Input: part model. Units: mm. Frame: model coordinates. Face numbers are marked on the shaded views. A direction names the side the tool comes from. Round coordinates to 2 decimals unless told otherwise and drop trailing zeros. Loops run counter-clockwise (first coordinate to the right, second up) from the corner with the lowest first, then second, coordinate; pieces in that order, holes last. Notation, with made-up numbers: (18.5, -19) -> (42.5, -19) arc R23 cw to (42.5, -8) -> close; hole circle Ø1 at (-39.5, 25). An arc over 180 degrees is marked (long way). One line per question, with ' | ' between items. Start each with the question number.
Q1. Material intervals for L1, parallel to X at y = 0, z = 32.1; L2, parallel to X at y = 0, z = 27.5; L3, parallel to X at y = 3.25, z = 28, sorted ascending.
Q2. Mould query, pull axis X, two halves, no side actions, for the marked faces 4, 5 and 6. Classes: pulls with the +X half, pulls with the -X half, needs draft (parallel to the pull), parting line crosses it, or undercut.
Q3. Contact query for flat-ended pins moving along their axis: P1, Ø9, axis at x = -34, y = 1.5, coming from the -Z side; P2, Ø6, axis at y = 3.5, z = 11, coming from the -X side; P3, Ø1, axis at x = 8.5, y = -0.5, coming from the +Z side; P4, Ø4, axis at x = -30.5, z = 19.5, coming from the +Y side. Output: stop coordinate, or through.
Q4. Access query for the marked faces 1, 2 and 3. Directions: +Z, -Z, +X, -X, +Y, -Y. A direction counts if a zero-diameter tool reaches every point of the face in a straight line with its end or side. Return the directions, or none.
Q5. Cut plane A-A on y = -5. Return loops of the section in (x, z), and give its area (3 significant figures).
Q6. Cut plane B-B on z = 14.5. Return loops of the section in (x, y), and give its area (3 significant figures).
Q7. Cut plane C-C on y = 0. State how many separate pieces and enclosed holes the cut face has, and give its area (3 significant figures).
Autodesk Inventor part; units mm, degrees
ref_plane "YZ Plane" through (0, 0, 0) normal (1, 0, 0) x (0, 1, 0)
ref_plane "XZ Plane" through (0, 0, 0) normal (0, 1, 0) x (-1, 0, 0)
ref_plane "XY Plane" through (0, 0, 0) normal (0, 0, 1) x (1, 0, 0)
sketch "Sketch1" plane through (0, 0, 0) normal (0, 0, 1) x (1, 0, 0)
  line L0 (-38.9875, 7.874) -> (38.9875, 7.874)
  line L1 (38.9875, 7.874) -> (38.9875, -7.874)
  line L2 (38.9875, -7.874) -> (-38.9875, -7.874)
  line L3 (-38.9875, -7.874) -> (-38.9875, 7.874)
  point P0 (0, 0)
  dimension "d2" = 77.975
  dimension "d3" = 38.9875
  dimension "d6" = 15.748
  dimension "d7" = 7.874
extrude "Extrusion1" add sketch "Sketch1" along normal blind 33.1075
sketch "Sketch2" plane through (0, 0, 0) normal (0, 0, -1) x (-1, 0, 0)
  line L0 (38.9875, 7.874) -> (38.9875, -7.874)
  line L1 (-38.9875, -7.874) -> (-38.9875, 7.874)
  line L2 (38.9875, -7.874) -> (-38.9875, -7.874)
  line L3 (-38.9875, 7.874) -> (38.9875, 7.874)
  line L4 (38.9875, -7.874) -> (26.9875, -7.874)
  line L5 (26.9875, -7.874) -> (26.9875, 7.874)
  line L6 (26.9875, 7.874) -> (38.9875, 7.874)
  line L7 (38.9875, 7.874) -> (38.9875, -7.874)
  line L8 (-38.9875, -7.874) -> (-26.9875, -7.874)
  line L9 (-26.9875, -7.874) -> (-26.9875, 7.874)
  line L10 (-26.9875, 7.874) -> (-38.9875, 7.874)
  line L11 (-38.9875, 7.874) -> (-38.9875, -7.874)
  line L12 (38.9875, -7.874) -> (-38.9875, -7.874)
  line L13 (12.0525, -7.874) -> (-14.5415, -7.874)
  line L14 (-14.5415, -7.874) -> (-14.5415, 7.874)
  line L15 (-14.5415, 7.874) -> (12.0525, 7.874)
  line L16 (12.0525, 7.874) -> (12.0525, -7.874)
  line L17 (26.9875, -7.874) -> (12.0525, -7.874)
  line L18 (12.0525, -7.874) -> (12.0525, 7.874)
  line L19 (12.0525, 7.874) -> (26.9875, 7.874)
  line L20 (26.9875, 7.874) -> (26.9875, -7.874)
  line L21 (-14.5415, -7.874) -> (-26.9875, -7.874)
  line L22 (-26.9875, -7.874) -> (-26.9875, 7.874)
  line L23 (-26.9875, 7.874) -> (-14.5415, 7.874)
  line L24 (-14.5415, 7.874) -> (-14.5415, -7.874)
  line L25 (26.9875, -7.874) -> (24.9875, -7.874)
  line L26 (24.9875, -7.874) -> (24.9875, 7.874)
  line L27 (24.9875, 7.874) -> (26.9875, 7.874)
  line L28 (26.9875, 7.874) -> (26.9875, -7.874)
  line L29 (-26.9875, -7.874) -> (-24.9875, -7.874)
  line L30 (-24.9875, -7.874) -> (-24.9875, 7.874)
  line L31 (-24.9875, 7.874) -> (-26.9875, 7.874)
  line L32 (-26.9875, 7.874) -> (-26.9875, -7.874)
  point P0 (0, 0)
  point P1 (38.9875, 0)
  point P2 (-38.9875, 0)
  point P3 (-1.5875, 0)
  point P4 (32.9875, 0)
  point P5 (-32.9875, 0)
  point P6 (-14.5415, -7.874)
  point P7 (-24.9875, 7.874)
  point P8 (24.9875, 7.874)
  dimension "d4" = 0
  dimension "d5" = 0
  dimension "d8" = 12
  dimension "d9" = 12
  dimension "d14" = 6
  dimension "d15" = 15.748
  dimension "d16" = 7.874
  dimension "d17" = 6
  dimension "d18" = 7.874
  dimension "d19" = 12.954
  dimension "d20" = 13.64
  dimension "d72" = 25.4
  dimension "d74" = 7.874
  dimension "d83" = 2
  dimension "d84" = 2
hole "Hole1" at (-32.9875, 0, 0) at (32.9875, 0, 0) direction (0, 0, 1) diameter 4.5 end through all counterbore diameter 8 counterbore depth 30.11
sketch "Sketch4" plane through (0, 0, 33.1075) normal (0, 0, 1) x (1, 0, 0)
  line L0 (38.9875, 7.874) -> (38.9875, -7.874)
  line L1 (-38.9875, -7.874) -> (-38.9875, 7.874)
  line L2 (38.9875, -7.874) -> (-38.9875, -7.874)
  line L3 (-38.9875, 7.874) -> (38.9875, 7.874)
  line L4 (38.9875, -7.874) -> (26.9875, -7.874)
  line L5 (26.9875, -7.874) -> (26.9875, 7.874)
  line L6 (26.9875, 7.874) -> (38.9875, 7.874)
  line L7 (38.9875, 7.874) -> (38.9875, -7.874)
  line L8 (-38.9875, -7.874) -> (-26.9875, -7.874)
  line L9 (-26.9875, -7.874) -> (-26.9875, 7.874)
  line L10 (-26.9875, 7.874) -> (-38.9875, 7.874)
  line L11 (-38.9875, 7.874) -> (-38.9875, -7.874)
  line L12 (38.9875, -7.874) -> (-38.9875, -7.874)
  line L13 (14.5415, -7.874) -> (-12.0525, -7.874)
  line L14 (-12.0525, -7.874) -> (-12.0525, 7.874)
  line L15 (-12.0525, 7.874) -> (14.5415, 7.874)
  line L16 (14.5415, 7.874) -> (14.5415, -7.874)
  line L17 (26.9875, -7.874) -> (14.5415, -7.874)
  line L18 (14.5415, -7.874) -> (14.5415, 7.874)
  line L19 (14.5415, 7.874) -> (26.9875, 7.874)
  line L20 (26.9875, 7.874) -> (26.9875, -7.874)
  line L21 (-12.0525, -7.874) -> (-26.9875, -7.874)
  line L22 (-26.9875, -7.874) -> (-26.9875, 7.874)
  line L23 (-26.9875, 7.874) -> (-12.0525, 7.874)
  line L24 (-12.0525, 7.874) -> (-12.0525, -7.874)
  point P0 (0, 0)
  point P1 (0, 0)
  point P2 (0, 0)
  point P3 (38.9875, 0)
  point P4 (-38.9875, 0)
  point P5 (1.5875, 0.076)
  point P6 (32.9875, 0)
  point P7 (-32.9875, 0)
  dimension "d48" = 0
  dimension "d49" = 0
  dimension "d50" = 12
  dimension "d51" = 12
  dimension "d54" = 6
  dimension "d55" = 15.748
  dimension "d56" = 7.874
  dimension "d57" = 6
  dimension "d58" = 7.874
  dimension "d59" = 13.64
  dimension "d60" = 12.954
  dimension "d61" = 25.4
  dimension "d75" = 7.95
hole "Hole3" [suppressed]
extrude "Extrusion2" cut sketch "Sketch2" against normal blind 4.508 contours L5 L2 L26 L3 | L26 L2 L16 L3 | L14 L2 L30 L3 | L30 L2 L9 L3
fillet "Fillet1" radius 2 2 edges at (-12.0525, 0, 0) (14.5415, 0, 0)
fillet "Fillet2" radius 2 2 edges at (-12.0525, 0, 4.508) (14.5415, 0, 4.508)
extrude "Extrusion3" cut sketch "Sketch2" against normal blind 23.11 contours L0 L2 L5 L3 | L5 L2 L26 L3 | L30 L2 L9 L3 | L9 L2 L1 L3
chamfer "Chamfer1" distance 2 angle 45 4 edges at (-38.9875, 7.874, 28.1088) (-38.9875, -7.874, 28.1088) (38.9875, 7.874, 28.1088) (38.9875, -7.874, 28.1088)
fillet "Fillet4" radius 2 4 edges at (-24.9875, 0, 4.508) (-24.9875, 0, 23.11) (24.9875, 0, 4.508) (24.9875, 0, 23.11)
sketch "Sketch5" plane through (-10.0525, -7.874, 0) normal (0, -1, 0) x (1, 0, 0)
  line L0 (13.89, 2.9975) -> (9.39, 2.9975)
  line L1 (-26.935, 33.1075) -> (47.04, 33.1075)
  circle A0 centre (11.64, 45.4575) radius 12.7
  point P0 (10.0525, 0)
  point P1 (11.64, 2.9975)
  point P2 (11.64, 33.1075)
  point P3 (14.601, 33.1075)
  point P4 (8.679, 33.1075)
  dimension "d86" = 25.4
  dimension "d87" = 12.35
extrude "Extrusion4" cut sketch "Sketch5" against normal through all contours L1 A0 picked at (11.9717, 33.0038)
sketch "Sketch6" plane through (0, 0, 33.1075) normal (0, 0, 1) x (1, 0, 0)
  line L0 (9.5855, 0) -> (8.5895, 0) construction
  line L1 (9.5855, 1.05) -> (8.5895, 1.05)
  line L2 (8.5895, -1.05) -> (9.5855, -1.05)
  arc A0 (9.5855, -1.05) -> (9.5855, 1.05) centre (9.5855, 0) ccw
  arc A1 (8.5895, 1.05) -> (8.5895, -1.05) centre (8.5895, 0) ccw
  line L3 (-12.0525, 7.874) -> (-12.0525, -7.874)
  line L4 (4.5485, -7.874) -> (-1.3735, -7.874)
  point P0 (0, 0)
  point P1 (1.5875, -5.5)
  point P2 (1.5875, 0)
  point P3 (-5.9125, 0)
  point P4 (9.0875, 0)
  dimension "d90" = 0
  dimension "d91" = 5.5
  dimension "d92" = 0
  dimension "d93" = 7.5
  dimension "d94" = 0
  dimension "d95" = 7.5
  dimension "d96" = 1.05
  dimension "d97" = 0.996
  dimension "d98" = 13.64
  dimension "d99" = 7.874
hole "Hole4" at (-5.9125, 0, 33.1075) direction (0, 0, -1) diameter 2.1 depth 2.1
sketch "Sketch8" plane through (0, 0, 33.1075) normal (0, 0, 1) x (1, 0, 0)
  line L0 (9.5855, 0) -> (8.5895, 0) construction
  line L1 (9.5855, 1.05) -> (8.5895, 1.05)
  line L2 (8.5895, -1.05) -> (9.5855, -1.05)
  arc A0 (9.5855, -1.05) -> (9.5855, 1.05) centre (9.5855, 0) ccw
  arc A1 (8.5895, 1.05) -> (8.5895, -1.05) centre (8.5895, 0) ccw
  line L3 (-12.0525, 7.874) -> (-12.0525, -7.874)
  line L4 (4.5485, -7.798) -> (-1.3735, -7.798)
  line L5 (4.5485, -7.874) -> (-1.3735, -7.874)
  point P0 (0, 0)
  point P1 (0, 0)
  point P2 (1.5875, -5.5)
  point P3 (1.5875, 0)
  point P4 (-5.9125, 0)
  point P5 (9.0875, 0)
  dimension "d121" = 0
  dimension "d122" = 5.5
  dimension "d123" = 0
  dimension "d124" = 7.5
  dimension "d125" = 0
  dimension "d126" = 7.5
  dimension "d127" = 1.05
  dimension "d128" = 0.996
  dimension "d129" = 13.64
  dimension "d157" = 7.874
extrude "Extrusion6" cut sketch "Sketch8" against normal blind 2.1
sketch "Sketch9" plane through (0, 0, 0) normal (0, 0, -1) x (-1, 0, 0)
  line L0 (38.9875, 7.874) -> (38.9875, -7.874)
  line L1 (-38.9875, -7.874) -> (-38.9875, 7.874)
  line L2 (38.9875, -7.874) -> (-38.9875, -7.874)
  line L3 (-38.9875, 7.874) -> (38.9875, 7.874)
  line L4 (38.9875, -7.874) -> (26.9875, -7.874)
  line L5 (26.9875, -7.874) -> (26.9875, 7.874)
  line L6 (26.9875, 7.874) -> (38.9875, 7.874)
  line L7 (38.9875, 7.874) -> (38.9875, -7.874)
  line L8 (-38.9875, -7.874) -> (-26.9875, -7.874)
  line L9 (-26.9875, -7.874) -> (-26.9875, 7.874)
  line L10 (-26.9875, 7.874) -> (-38.9875, 7.874)
  line L11 (-38.9875, 7.874) -> (-38.9875, -7.874)
  line L12 (38.9875, -7.874) -> (-38.9875, -7.874)
  line L13 (12.0525, -7.874) -> (-14.5415, -7.874)
  line L14 (-14.5415, -7.874) -> (-14.5415, 7.874)
  line L15 (-14.5415, 7.874) -> (12.0525, 7.874)
  line L16 (12.0525, 7.874) -> (12.0525, -7.874)
  line L17 (26.9875, -7.874) -> (12.0525, -7.874)
  line L18 (12.0525, -7.874) -> (12.0525, 7.874)
  line L19 (12.0525, 7.874) -> (26.9875, 7.874)
  line L20 (26.9875, 7.874) -> (26.9875, -7.874)
  line L21 (-14.5415, -7.874) -> (-26.9875, -7.874)
  line L22 (-26.9875, -7.874) -> (-26.9875, 7.874)
  line L23 (-26.9875, 7.874) -> (-14.5415, 7.874)
  line L24 (-14.5415, 7.874) -> (-14.5415, -7.874)
  line L25 (26.9875, -7.874) -> (24.9875, -7.874)
  line L26 (24.9875, -7.874) -> (24.9875, 7.874)
  line L27 (24.9875, 7.874) -> (26.9875, 7.874)
  line L28 (26.9875, 7.874) -> (26.9875, -7.874)
  line L29 (-26.9875, -7.874) -> (-24.9875, -7.874)
  line L30 (-24.9875, -7.874) -> (-24.9875, 7.874)
  line L31 (-24.9875, 7.874) -> (-26.9875, 7.874)
  line L32 (-26.9875, 7.874) -> (-26.9875, -7.874)
  point P0 (0, 0)
  point P1 (0, 0)
  point P2 (38.9875, 0)
  point P3 (-38.9875, 0)
  point P4 (-1.5875, 0.076)
  point P5 (32.9875, 0)
  point P6 (-32.9875, 0)
  point P7 (-14.5415, -7.874)
  point P8 (-24.9875, 7.874)
  point P9 (24.9875, 7.874)
  dimension "d135" = 0
  dimension "d136" = 0
  dimension "d137" = 12
  dimension "d138" = 12
  dimension "d139" = 6
  dimension "d140" = 15.748
  dimension "d141" = 7.874
  dimension "d142" = 6
  dimension "d143" = 7.874
  dimension "d144" = 12.954
  dimension "d145" = 13.64
  dimension "d146" = 25.4
  dimension "d147" = 7.95
  dimension "d148" = 2
  dimension "d149" = 2
hole "Hole5" at (1.5875, 0.076, 0) direction (0, 0, 1) diameter 3.302 depth 12.3
properties part number "ADAPTER_new-focus-8821"
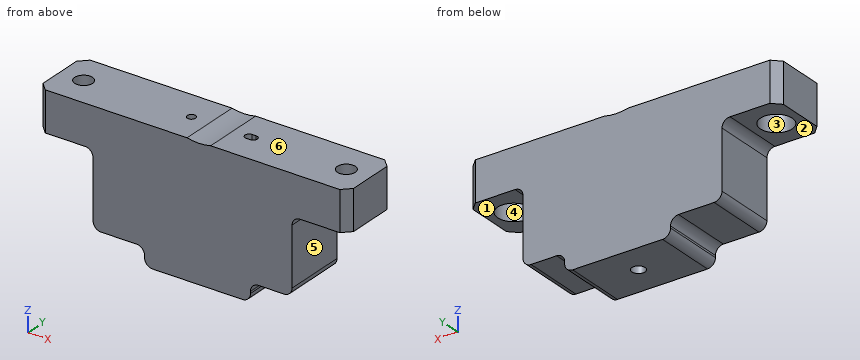
Results:
1) L1: -38.99 to -35.24, -30.74 to -6.96, -4.86 to 7.54, 10.64 to 30.74, 35.24 to 38.99 | L2: -38.99 to -36.99, -28.99 to 28.99, 36.99 to 38.99 | L3: -38.99 to -35.32, -30.66 to 30.66, 35.32 to 38.99
2) face 4: undercut | face 5: pulls with the +X half | face 6: needs draft
3) P1: z = 23.11 | P2: x = -24.99 | P3: z = 31.01 | P4: through
4) face 1: -Z, +X, +Y, -Y | face 2: -Z, -X, +Y, -Y | face 3: -Z
5) outline: (-38.99, 23.11) -> (-26.99, 23.11) arc R2 cw to (-24.99, 21.11) -> (-24.99, 6.51) arc R2 ccw to (-22.99, 4.51) -> (-14.05, 4.51) arc R2 cw to (-12.05, 2.51) -> (-12.05, 2) arc R2 ccw to (-10.05, 0) -> (12.54, 0) arc R2 ccw to (14.54, 2) -> (14.54, 2.51) arc R2 cw to (16.54, 4.51) -> (22.99, 4.51) arc R2 ccw to (24.99, 6.51) -> (24.99, 21.11) arc R2 cw to (26.99, 23.11) -> (38.99, 23.11) -> (38.99, 33.11) -> (4.55, 33.11) arc R12.7 cw to (-1.37, 33.11) -> (-38.99, 33.11) -> close | area: 1,830 mm^2
6) outline: (-24.99, -7.87) -> (24.99, -7.87) -> (24.99, 7.87) -> (-24.99, 7.87) -> close | area: 787 mm^2
7) separate pieces: 3 | enclosed holes: 0 | area: 1,640 mm^2
